The listing builds one solid part. Answer for the finished solid, in the listing's coordinates (mm). Coordinates: 2 decimals unless noted, no trailing zeros. Loops run counter-clockwise (first coordinate to the right, second up) from the corner with the lowest first, then second, coordinate; pieces in that order, holes last. Notation, with made-up numbers: (-30, 32) - (4, 32) arc R15 ccw to (4, 51) - close; hole circle Ø10 at (-37, 19). An arc over 180 degrees is marked (long way). Use one line per item in the form item = value. Start each with the question number.
```python
from build123d import *

# Parameters (mm, degrees)
EXTRUDE1_DEPTH        = 1
SKETCH2_W             = 165
SKETCH2_H             = 32
CUT_EXTRUDE1_DEPTH    = 1
SKETCH3_R             = 6.5
SKETCH3_R_2           = 5.25
CORTE_EXTRUS_O1_DEPTH = 2


with BuildPart() as part:
    # Sketch1 → Extrude1 (new body)
    with BuildSketch(Plane.XY):
        Polygon((-115, 75), (115, 75), (115, 60), (130, 60), (130, -60), (115, -60), (115, -75), (-115, -75), (-115, -60), (-130, -60), (-130, 60), (-115, 60), align=None)
    extrude(amount=EXTRUDE1_DEPTH)

    # Sketch2 → Cut-Extrude1 (cut)
    with BuildSketch(Plane.XY.offset(1)):
        with Locations((-7.5, 28.75)):
            Rectangle(SKETCH2_W, SKETCH2_H)
    extrude(amount=-CUT_EXTRUDE1_DEPTH, mode=Mode.SUBTRACT)

    # Sketch3 → Corte-extrusão1 (cut, through all)
    with BuildSketch(Plane.XY.offset(1)):
        with Locations((-113.5, 53.5)):
            Circle(SKETCH3_R)
        with Locations((-113.5, 28.75)):
            Circle(SKETCH3_R)
        with Locations((-56.5, 3.5)):
            Circle(SKETCH3_R)
        with Locations((-5.5, 3.5)):
            Circle(SKETCH3_R)
        with Locations((45.5, 3.5)):
            Circle(SKETCH3_R)
        with Locations((45.5, 53.5)):
            Circle(SKETCH3_R)
        with Locations((-5.5, 53.5)):
            Circle(SKETCH3_R)
        with Locations((-56.5, 53.5)):
            Circle(SKETCH3_R)
        with Locations((96.5, 35)):
            Circle(SKETCH3_R_2)
        with Locations((109.5, 35)):
            Circle(SKETCH3_R_2)
        with Locations((109.5, 22)):
            Circle(SKETCH3_R_2)
        with Locations((96.5, 22)):
            Circle(SKETCH3_R_2)
    extrude(amount=-CORTE_EXTRUS_O1_DEPTH, mode=Mode.SUBTRACT)


solid = part.part
```
(1) A cutting plane is placed at D-D (x = 45.5). Determine the outline of the cut face in (y, z), then the cut area to 3 significant figures.
(2) A cutting plane is placed at C-C (z = 0.45). State how many separate pieces and enclosed holes the cut face has, then the cut area to 3 significant figures.
(3) Determine the mould class of faces 1 (the face through (44.091, 47.155, 0.507)), 2 (the face through (2, 1, 0)), 3 (the face through (-6.909, 47.155, 0.507)) for opening direction X: +X half, -X half, draft (parallel to the pull), parting line (faces both ways), or undercut.
(4) A cutting plane is placed at B-B (y = 3.5). Determine the outline of the cut face in (x, z), then the cut area to 3 significant figures.
(5) Find the intervals of material crossed by probe 1 along Y at (x, z) = (-56.5, 0.7); probe 2 along Y at (x, z) = (96.5, 0.4); probe 3 along Y at (x, z) = (-75, 0.9), in increasing order. Write a range as from..to.
(6) This flat-tipped pin is pushed along its axis until it touches: pin 1 Ø0.5 at (x, z) = (-121.5, 0.5) entering from +Y. Where does it stop, or does it pass through?
(7) A cutting plane is placed at A-A (x = 96.5). Determine the outline of the cut face in (y, z), then the cut area to 3 significant figures.
Evaluation:
q1.outline = (-75, 0) - (-3, 0) - (-3, 1) - (-75, 1) - close; (10, 0) - (12.75, 0) - (12.75, 1) - (10, 1) - close; (44.75, 0) - (47, 0) - (47, 1) - (44.75, 1) - close; (60, 0) - (75, 0) - (75, 1) - (60, 1) - close
q1.area = 92.0 mm^2
q2.separate_pieces = 1
q2.enclosed_holes = 13
q2.area = 31,400 mm^2
q3.face_1 = undercut
q3.face_2 = draft
q3.face_3 = undercut
q4.outline = (-130, 0) - (-63, 0) - (-63, 1) - (-130, 1) - close; (-50, 0) - (-12, 0) - (-12, 1) - (-50, 1) - close; (1, 0) - (39, 0) - (39, 1) - (1, 1) - close; (52, 0) - (130, 0) - (130, 1) - (52, 1) - close
q4.area = 221 mm^2
q5.probe_1 = -75..-3, 10..12.75, 44.75..47, 60..75
q5.probe_2 = -75..16.75, 27.25..29.75, 40.25..75
q5.probe_3 = -75..12.75, 44.75..75
q6.pin_1 = 60
q7.outline = (-75, 0) - (16.75, 0) - (16.75, 1) - (-75, 1) - close; (27.25, 0) - (29.75, 0) - (29.75, 1) - (27.25, 1) - close; (40.25, 0) - (75, 0) - (75, 1) - (40.25, 1) - close
q7.area = 129 mm^2
